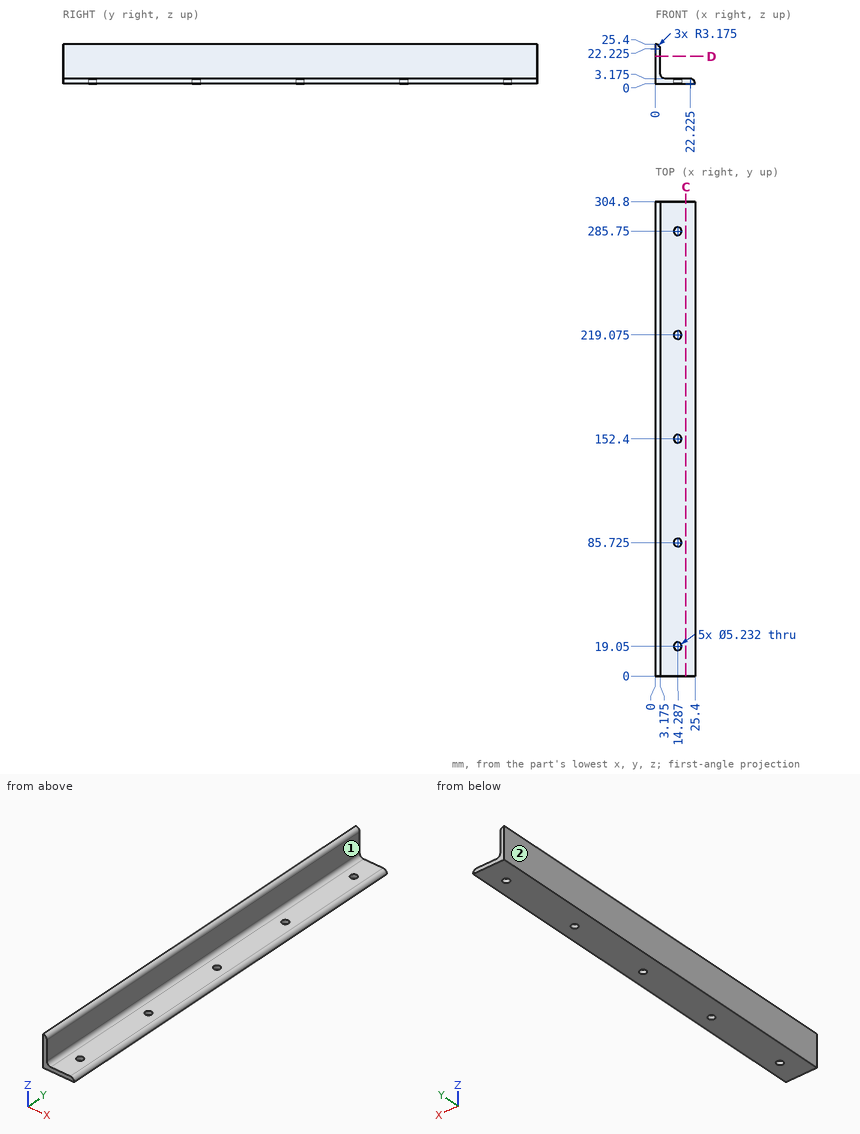
Answer from the drawing. Dimensions are ordinates in mm from the lowest x, y and z of the part. A direction names the side the tool comes from. Give positions to 0.01 mm unless a question says otherwise; leave off trailing zeros. Write each loop counter-clockwise with the first axis right and the second up, starting at its lowest first coordinate (ties: lowest second). Pieces come first, ordered by that corner, then holes. Notation, with made-up numbers: (-15.75, 39) - (12.25, 39) arc R22 ccw to (12.25, 57) - close; hole circle Ø2 at (-1.5, 68.5). An arc over 180 degrees is marked (long way). One line per item, written item: value. Start each with the question number.
1. Consider probe 1 along X at (y, z) = (69.5, 12) (1 decimal); probe 2 along Z at (x, y) = (23.5, 244). Determine where each line is inside the solid, lowest interval first.
2. Find section D-D (z = 17.5). Write down the section's boundary in (x, y) (1 decimal).
3. Find section C-C (x = 19.5). Write down the section's boundary in (y, z) (1 decimal).
4. For the marked faces 1 and 2, determine the directions among +Z, -Z, +X, -X, +Y, -Y from which every point of the face is accessible in a straight line to the end or side of a thin tool.
5. Given pin 1 (8 mm diameter, centred on y = 103, z = 17, fed in from +X) (1 decimal); pin 2 (10 mm diameter, centred on x = 8.5, z = 18.5, fed in from -Y); pin 3 (7 mm diameter, centred on x = 14.29, y = 219.08, fed in from +Z) (1 decimal); pin 4 (4 mm diameter, centred on y = 36, z = 4.5, fed in from +X), each flat-ended and moving along its own axis, determine where each tip first touches the part or whether it passes through.
Geometry results:
1. probe 1: 0 to 3.2
1. probe 2: 0 to 2.91
2. outline: (0, 0) - (3.2, 0) - (3.2, 304.8) - (0, 304.8) - close
3. outline: (0, 0) - (304.8, 0) - (304.8, 3.2) - (0, 3.2) - close
4. face 1: +Z, +X, +Y, -Y
4. face 2: +Z, -Z, -X, +Y, -Y
5. pin 1: x = 3.2
5. pin 2: through
5. pin 3: z = 3.2
5. pin 4: x = 24.18
